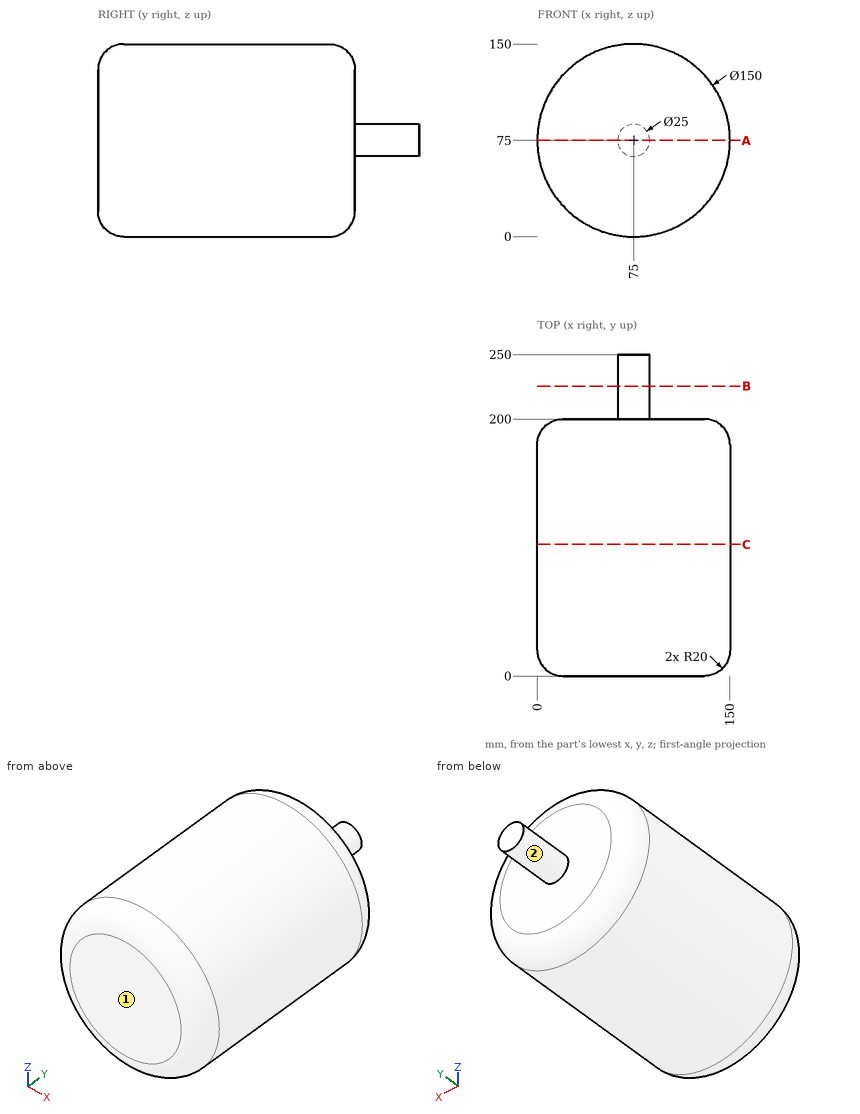
Geometry: see drawing. Coordinates: mm, zero at the bounding-box minimum. A direction names the side the tool comes from. Give positions to 0.01 mm unless a question says otherwise; leave off trailing zeros. Loops run counter-clockwise (first coordinate to the right, second up) from the corner with the lowest first, then second, coordinate; pieces in that order, holes last. Notation, with made-up numbers: (-32, 58.5) -> (-7, 58.5) arc R24 cw to (-7, 68.5) -> close; hole circle Ø11 at (44, 56). An arc over 180 degrees is marked (long way). Put each result on its own line as item: value.
1. Cut plane A-A (z = 75). Return the cut outline in (x, y), plus the area to 3 significant figures.
Taken from the geometry:
outline: (0, 20) arc R20 ccw to (20, 0) -> (130, 0) arc R20 ccw to (150, 20) -> (150, 180) arc R20 ccw to (130, 200) -> (87.5, 200) -> (87.5, 250) -> (62.5, 250) -> (62.5, 200) -> (20, 200) arc R20 ccw to (0, 180) -> close
area: 30,900 mm2
2. Cut plane B-B (y = 225.5). Return the cut outline in (x, z).
Taken from the geometry:
outline: circle Ø25 at (75, 75)
3. Set-up query: the marked faces 1 and 2. Return all of +Z, -Z, +X, -X, +Y, -Y with unobstructed straight access to the full face (end or side cutting, diameter ignored); none if empty.
Taken from the geometry:
face 1: +Z, -Z, +X, -X, -Y
face 2: +Y
4. Pin query (flat end, axial travel): P1, Ø3, axis at y = 152.5, z = 98.5, coming from the -X side; P2, Ø2, axis at x = 34.5, y = 91.5, coming from the -Z side; P3, Ø10, axis at x = 67, z = 126, coming from the +Y side. Return the tip coordinate at first contact, or that it passes through.
Taken from the geometry:
P1: stops at x = 3.3
P2: stops at z = 11.24
P3: stops at y = 200
5. Ray query, line 1 along Y through (x, z) = (123, 73); line 2 along Z through (x, y) = (106.5, 60); line 3 along X through (y, z) = (35, 8.5). Return the intervals inside material, ascending. Write a range as [from, to].
Taken from the geometry:
line 1: y = [0, 200]
line 2: z = [6.94, 143.06]
line 3: x = [40.32, 109.68]
6. Cut plane C-C (y = 102.5). Return the cut outline in (x, z).
Taken from the geometry:
outline: circle Ø150 at (75, 75)
